```python
from build123d import *

# Parameters (mm, degrees)
F1_DEPTH = 20
F2_DEPTH = 10
F3_W     = 55.5881783366
F3_H     = 43.1093648076
F4_DEPTH = 5


with BuildPart() as f1:
    # F0 (on Top) → F1 (new body)
    with BuildSketch(Plane.XY):
        with BuildLine():
            ThreePointArc((-38.2674500346, 0), (-52.9121109753, 35.3553390593), (-88.2674500346, 50))
            Line((-88.2674500346, 50), (-88.2674500346, 10))
            ThreePointArc((-88.2674500346, 10), (-81.1963822228, 7.0710678119), (-78.2674500346, 0))
            ThreePointArc((-78.2674500346, 0), (-81.1963822228, -7.0710678119), (-88.2674500346, -10))
            Line((-88.2674500346, -10), (-88.2674500346, -50))
            ThreePointArc((-88.2674500346, -50), (-52.9121109753, -35.3553390593), (-38.2674500346, 0))
        make_face()
        with BuildLine():
            Line((88.2674500346, 50), (-88.2674500346, 50))
            ThreePointArc((-88.2674500346, 50), (-52.9121109753, 35.3553390593), (-38.2674500346, 0))
            ThreePointArc((-38.2674500346, 0), (-52.9121109753, -35.3553390593), (-88.2674500346, -50))
            Line((-88.2674500346, -50), (88.2674500346, -50))
            Line((88.2674500346, -50), (88.2674500346, 50))
        make_face()
        with BuildLine():
            Line((-88.2674500346, 10), (-88.2674500346, 50))
            ThreePointArc((-88.2674500346, 50), (-138.2674500346, 0), (-88.2674500346, -50))
            Line((-88.2674500346, -50), (-88.2674500346, -10))
            ThreePointArc((-88.2674500346, -10), (-98.2674500346, 0), (-88.2674500346, 10))
        make_face()
    extrude(amount=F1_DEPTH)

    # F0 (on Top) → F2 (cut)
    with BuildSketch(Plane.XY):
        with BuildLine():
            Line((-88.2674500346, 10), (-88.2674500346, 50))
            ThreePointArc((-88.2674500346, 50), (-138.2674500346, 0), (-88.2674500346, -50))
            Line((-88.2674500346, -50), (-88.2674500346, -10))
            ThreePointArc((-88.2674500346, -10), (-98.2674500346, 0), (-88.2674500346, 10))
        make_face()
    extrude(amount=F2_DEPTH, mode=Mode.SUBTRACT)

    # F3 (on face) → F4 (cut)
    with BuildSketch(Plane.XY.offset(20)):
        Rectangle(F3_W, F3_H)
    extrude(amount=-F4_DEPTH, mode=Mode.SUBTRACT)


solid = f1.part
```
The listing builds one solid part. Answer for the finished solid, in the listing's coordinates (mm). A direction names the side the tool comes from. Coordinates: 2 decimals unless noted, no trailing zeros. Write each loop counter-clockwise with the first axis right and the second up, starting at its lowest first coordinate (ties: lowest second). Pieces come first, ordered by that corner, then holes.
Q1. Section B-B, the plane z = 5 is taken. Write down the section's boundary in (x, y), then the cut area to 3 significant figures.
Returned:
outline: (-88.27, -50) - (88.27, -50) - (88.27, 50) - (-88.27, 50) - (-88.27, 10) arc R10 cw to (-88.27, -10) - close
area: 17,500 mm2
Q2. Section A-A, the plane x = 13.5 is taken. Write down the section's boundary in (y, z).
Returned:
outline: (-50, 0) - (50, 0) - (50, 20) - (21.55, 20) - (21.55, 15) - (-21.55, 15) - (-21.55, 20) - (-50, 20) - close
Q3. The mould has two halves that part along X. Classify faces 1 (the flat face through (-27, 23, 20)), 2 (the flat face through (-88.267, 30, 5)), 3 (the flat face through (88.267, -1, 10)), 4 (the flat face through (27.794, 0, 18)): released by +X, released by -X, zero draft, split by the parting line, or undercut.
Returned:
face 1: zero draft
face 2: released by -X
face 3: released by +X
face 4: undercut
Q4. Find the intervals of material crossed by line 1 along X through (y, z) = (13, 1.25); line 2 along Z through (x, y) = (-111.5, 35.5); line 3 along X through (y, z) = (15, 10.5), in increasing order.
Returned:
line 1: x = -88.27 to 88.27
line 2: z = 10 to 20
line 3: x = -135.96 to 88.27
Q5. Section C-C, the plane y = -42 is taken. Write down the section's boundary in (x, z).
Returned:
outline: (-115.4, 10) - (-88.27, 10) - (-88.27, 0) - (88.27, 0) - (88.27, 20) - (-115.4, 20) - close
Q6. Given P1, Ø5, axis at y = 29.5, z = 3.5, coming from the -X side; P2, Ø1.5, axis at x = 53.5, y = 8.5, coming from the -Z side; P3, Ø2, axis at y = 13, z = 14.5, coming from the -X side; P4, Ø2.5, axis at y = 1, z = 18, coming from the -X side, each flat-ended and moving along its own axis, determine where each tip first touches the part or whether it passes through.
Returned:
P1: stops at x = -88.27
P2: stops at z = 0
P3: stops at x = -136.81
P4: stops at x = -138.27
Q7. Section D-D, the plane y = 25.5 is taken. Write down the section's boundary in (x, z).
Returned:
outline: (-131.28, 10) - (-88.27, 10) - (-88.27, 0) - (88.27, 0) - (88.27, 20) - (-131.28, 20) - close
Q8. Which of the six approach directions +Z, -Z, +X, -X, +Y, -Y give full straight-line access (tool end or side, diameter ignored) to faces 5 (the flat face through (1, 50, 10)), 6 (the flat face through (-27.794, 0, 18)), 7 (the flat face through (-108, 1, 10))?
Returned:
face 5: +Z, -Z, +X, -X, +Y
face 6: +Z
face 7: -Z, -X, +Y, -Y
